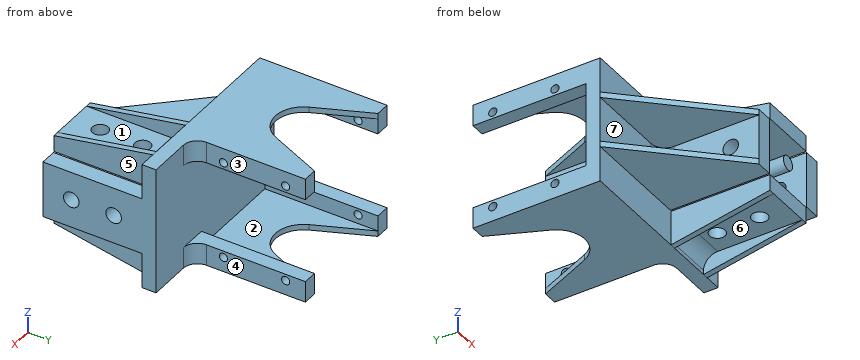
from build123d import *

# Parameters (mm, degrees)
BOSS_EXTRUDE1_DEPTH           = 45
SKETCH3_W                     = 30
SKETCH3_H                     = 40
CUT_EXTRUDE1_DEPTH            = 83.196411114
SKETCH4_W                     = 32
SKETCH4_H                     = 32
SKETCH4_W_2                   = 20.5
SKETCH4_H_2                   = 20.5
SKETCH4_R                     = 2.5
BOSS_EXTRUDE2_DEPTH           = 35
SKETCH6_W                     = 6
SKETCH6_H                     = 6
CUT_EXTRUDE4_DEPTH            = 35
RIB1_REACH                    = 84.092
SKETCH9_WALL_W                = 214.287640152
SKETCH9_WALL_H                = 2
LPATTERN1_COUNT               = 2
LPATTERN1_PITCH               = 18
RIB6_REACH                    = 95.874
SKETCH14_WALL_W               = 225.34562544
SKETCH14_WALL_H               = 2
RIB7_START                    = -2
RIB7_DEPTH                    = 2
CIRPATTERN3_START             = -9.75
CIRPATTERN3_DEPTH             = 2
CIRPATTERN3_START_2           = 8.25
CIRPATTERN3_2_DEPTH           = 2
FILLET2_R                     = 5
FILLET3_R                     = 5
RIB10_REACH                   = 89.794
SKETCH17_WALL_W               = 221.248919868
SKETCH17_WALL_H               = 2
RIB11_REACH                   = 89.794
SKETCH18_WALL_W               = 221.248919868
SKETCH18_WALL_H               = 2
FILLET4_R                     = 10
LPATTERN2_COUNT               = 2
LPATTERN2_PITCH               = 43
FILLET4_OF_LPATTERN2_R        = 10
M5_CLEARANCE_HOLE2_AT_2_COUNT = 2
M5_CLEARANCE_HOLE2_AT_2_PITCH = 15
CIRPATTERN4_START             = 6.5
CIRPATTERN4_OUTLINE_R         = 2.75
CIRPATTERN4_DEPTH             = 5.75
CIRPATTERN4_START_2           = -15.75
CIRPATTERN4_2_OUTLINE_R       = 2.75
CIRPATTERN4_2_DEPTH           = 5.75
CIRPATTERN4_START_3           = 10.5
CIRPATTERN4_3_OUTLINE_R       = 2.75
CIRPATTERN4_3_DEPTH           = 5.75
M2_5_CLEARANCE_HOLE1_D        = 2.9


# Read off the part's stored shape, not the designer's step: Rib7, CirPattern3, CirPattern4
with BuildPart() as part:
    # Sketch2 → Boss-Extrude1 (new body)
    with BuildSketch(Plane.XY):
        Polygon((-48.75, -22.5), (16.25, -22.5), (16.25, -17.5), (-3.75, -17.5), (-3.75, 22.5), (-8.75, 22.5), (-8.75, -17.5), (-43.75, -17.5), (-43.75, 22.5), (-48.75, 22.5), align=None)
    extrude(amount=BOSS_EXTRUDE1_DEPTH)

    # Sketch3 → Cut-Extrude1 (cut, through all)
    with BuildSketch(Plane(origin=(-48.75, 0, 0), x_dir=(0, 0, -1), z_dir=(1, 0, 0))):
        with Locations((-22.5, 2.5)):
            Rectangle(SKETCH3_W, SKETCH3_H)
    extrude(amount=CUT_EXTRUDE1_DEPTH, mode=Mode.SUBTRACT)

    # Sketch4 → Boss-Extrude2 (add)
    # profile 1 of 2: a face of its own
    with BuildSketch(Plane.XZ.offset(22.5)):
        with Locations((0.25, 22.5)):
            Rectangle(SKETCH4_W, SKETCH4_H)
        with Locations((0.25, 22.5)):
            Rectangle(SKETCH4_W_2, SKETCH4_H_2, mode=Mode.SUBTRACT)
    # profile 2 of 2: a face of its own
    with BuildSketch(Plane.XZ.offset(22.5)):
        with Locations(Location((0.25, 22.5, 0), (0, 0, 180))):
            Circle(SKETCH4_R)
    extrude(amount=BOSS_EXTRUDE2_DEPTH)

    # Sketch6 → Cut-Extrude4 (cut)
    with BuildSketch(Plane(origin=(0, -57.5, 0), x_dir=(-1, 0, 0), z_dir=(0, -1, 0))):
        with Locations((12.75, -35.5)):
            Rectangle(SKETCH6_W, SKETCH6_H)
        with Locations((-13.25, -35.5)):
            Rectangle(SKETCH6_W, SKETCH6_H)
        with Locations((-13.25, -9.5)):
            Rectangle(SKETCH6_W, SKETCH6_H)
        with Locations((12.75, -9.5)):
            Rectangle(SKETCH6_W, SKETCH6_H)
    extrude(amount=-CUT_EXTRUDE4_DEPTH, mode=Mode.SUBTRACT)

    # Sketch9 wall → Rib1 (add, up to next)
    with BuildSketch(Plane(origin=(-32.25, -40, 32.5), x_dir=(-0.686012868689, 0.727589406185, 0), z_dir=(-0.727589406185, -0.686012868689, 0)), mode=Mode.PRIVATE) as rib1_sk1:
        with Locations((0, 1)):
            Rectangle(SKETCH9_WALL_W, SKETCH9_WALL_H)
    rib1_tool1 = extrude(rib1_sk1.sketch, amount=-RIB1_REACH, mode=Mode.PRIVATE) - part.part
    rib1 = rib1_tool1.solids().sort_by_distance((-32.25, -40, 32.5))[0]
    add(rib1)

    # LPattern1: Rib1 ×2
    with Locations(*[(0, 0, -i * LPATTERN1_PITCH) for i in range(1, LPATTERN1_COUNT)]):
        add(rib1)

    # Sketch14 wall → Rib6 (add, up to next)
    with BuildSketch(Plane(origin=(10.25, -40, 3.25), x_dir=(0, 0.983188736076, -0.182592193843), z_dir=(0, 0.182592193843, 0.983188736076)), mode=Mode.PRIVATE) as rib6_sk1:
        with Locations((0, 1)):
            Rectangle(SKETCH14_WALL_W, SKETCH14_WALL_H)
    rib6_tool1 = extrude(rib6_sk1.sketch, amount=RIB6_REACH, mode=Mode.PRIVATE) - part.part
    add(rib6_tool1.solids().sort_by_distance((10.25, -40, 3.25))[0])

    # Rib7 outline → Rib7 (add)
    with BuildSketch(Plane.ZY.offset(9.75).offset(RIB7_START)):
        Polygon((0, -22.5), (6.5, -57.5), (6.5, -22.5), align=None)
    extrude(amount=RIB7_DEPTH)

    # CirPattern3 outline → CirPattern3 (add)
    with BuildSketch(Plane.YZ.offset(CIRPATTERN3_START)):
        Polygon((-22.5, 38.5), (-22.5, 45), (-57.5, 38.5), align=None)
    extrude(amount=CIRPATTERN3_DEPTH)

    # CirPattern3 2 outline → CirPattern3 2 (add)
    with BuildSketch(Plane.YZ.offset(CIRPATTERN3_START_2)):
        Polygon((-22.5, 38.5), (-22.5, 45), (-57.5, 38.5), align=None)
    extrude(amount=CIRPATTERN3_2_DEPTH)

    # Fillet2
    fillet2_edges = [part.edges().sort_by_distance(p)[0] for p in [
        (-15.75, -22.5, 22.5),
        (0.25, -22.5, 6.5),
        (0.25, -22.5, 38.5),
    ]]
    fillet(fillet2_edges, radius=FILLET2_R)

    # Fillet3
    fillet3_edges = [part.edges().sort_by_distance(p)[0] for p in [
        (-3.75, -17.5, 41.25),
        (-3.75, -17.5, 3.75),
    ]]
    fillet(fillet3_edges, radius=FILLET3_R)

    # Sketch17 wall → Rib10 (add, up to next)
    with BuildSketch(Plane(origin=(-35, 2.5, 45), x_dir=(0.40081883402, -0.916157334902, 0), z_dir=(0.916157334902, 0.40081883402, 0)), mode=Mode.PRIVATE) as rib10_sk1:
        with Locations((0, 1)):
            Rectangle(SKETCH17_WALL_W, SKETCH17_WALL_H)
    rib10_tool1 = extrude(rib10_sk1.sketch, amount=-RIB10_REACH, mode=Mode.PRIVATE) - part.part
    rib10 = rib10_tool1.solids().sort_by_distance((-35, 2.5, 45))[0]
    add(rib10)

    # Sketch18 wall → Rib11 (add, up to next)
    with BuildSketch(Plane(origin=(-17.5, 2.5, 45), x_dir=(0.40081883402, 0.916157334902, 0), z_dir=(-0.916157334902, 0.40081883402, 0)), mode=Mode.PRIVATE) as rib11_sk1:
        with Locations((0, 1)):
            Rectangle(SKETCH18_WALL_W, SKETCH18_WALL_H)
    rib11_tool1 = extrude(rib11_sk1.sketch, amount=-RIB11_REACH, mode=Mode.PRIVATE) - part.part
    rib11 = rib11_tool1.solids().sort_by_distance((-17.5, 2.5, 45))[0]
    add(rib11)

    # Fillet4
    # the kernel refuses this fillet: 10 mm, written as the material it adds along each edge
    with BuildSketch(Plane(origin=(-26.25, -17.5, 45), x_dir=(-0.4008188340200225, 0.9161573349020514, 0), z_dir=(0, 0, -1))) as fillet4_piece_1:
        with BuildLine():
            CenterArc((FILLET4_R * 2.28571428571, FILLET4_R), FILLET4_R, 137.258755461, 132.741244539)
            Line((FILLET4_R * 1.55128805621, FILLET4_R * 1.67868852459), (0, 0))
            Line((0, 0), (FILLET4_R * 2.28571428571, 0))
        make_face()
    extrude(amount=2)

    # LPattern2: Rib10, Rib11 ×2
    with Locations(*[(0, 0, -i * LPATTERN2_PITCH) for i in range(1, LPATTERN2_COUNT)]):
        add(rib10)
        add(rib11)

    # Fillet4 of LPattern2
    # the kernel refuses this fillet: 10 mm, written as the material it adds along each edge
    with BuildSketch(Plane(origin=(-26.25, -17.5, 59.142857143), x_dir=(-0.4008188340200225, 0.9161573349020515, 0), z_dir=(0, 0, -1))) as fillet4_of_lpattern2_piece_1_section:
        with BuildLine():
            CenterArc((FILLET4_OF_LPATTERN2_R * 2.28571428571, FILLET4_OF_LPATTERN2_R), FILLET4_OF_LPATTERN2_R, 137.258755461, 132.741244539)
            Line((FILLET4_OF_LPATTERN2_R * 1.5512880562, FILLET4_OF_LPATTERN2_R * 1.67868852459), (0, 0))
            Line((0, 0), (FILLET4_OF_LPATTERN2_R * 2.28571428571, 0))
        make_face()
    fillet4_of_lpattern2_piece_1 = extrude(amount=59.142857143, mode=Mode.PRIVATE)
    fillet4_of_lpattern2_piece_1 = split(fillet4_of_lpattern2_piece_1, bisect_by=Plane(origin=(-26.25, -6.732617491, 43), z_dir=(0, 0, 1)), keep=Keep.TOP, mode=Mode.PRIVATE)
    fillet4_of_lpattern2_piece_1 = split(fillet4_of_lpattern2_piece_1, bisect_by=Plane(origin=(-26.25, -6.732617491, 45), z_dir=(0, 0, -1)), keep=Keep.TOP, mode=Mode.PRIVATE)
    add(fillet4_of_lpattern2_piece_1)
    with BuildSketch(Plane(origin=(-26.25, -17.5, 2), x_dir=(-0.4008188340200225, 0.9161573349020514, 0), z_dir=(0, 0, -1))) as fillet4_of_lpattern2_piece_2:
        with BuildLine():
            CenterArc((FILLET4_OF_LPATTERN2_R * 2.28571428571, FILLET4_OF_LPATTERN2_R), FILLET4_OF_LPATTERN2_R, 137.258755461, 132.741244539)
            Line((FILLET4_OF_LPATTERN2_R * 1.55128805621, FILLET4_OF_LPATTERN2_R * 1.67868852459), (0, 0))
            Line((0, 0), (FILLET4_OF_LPATTERN2_R * 2.28571428571, 0))
        make_face()
    extrude(amount=2)

    # Sketch22 → M5 Clearance Hole2 (revolve, cut)
    with BuildSketch(Plane(origin=(0.25, -32.5, 38.5), x_dir=(0, -1, 0), z_dir=(1, 0, 0))):
        Polygon((0, 0), (0, 7.652366702), (2.75, 6), (2.75, 0), align=None)
    m5_clearance_hole2 = revolve(axis=Axis((0.25, -32.5, 44.85), (0, 0, -1)), mode=Mode.SUBTRACT)

    # M5 Clearance Hole2 at 2: M5 Clearance Hole2 ×2
    with Locations(*[(0, -i * M5_CLEARANCE_HOLE2_AT_2_PITCH, 0) for i in range(1, M5_CLEARANCE_HOLE2_AT_2_COUNT)]):
        add(m5_clearance_hole2, mode=Mode.SUBTRACT)

    # CirPattern4 outline → CirPattern4 (cut)
    with BuildSketch(Plane.XY.offset(CIRPATTERN4_START)):
        with Locations((0.25, -47.5)):
            Circle(CIRPATTERN4_OUTLINE_R)
        with Locations((0.25, -32.5)):
            Circle(CIRPATTERN4_OUTLINE_R)
    extrude(amount=CIRPATTERN4_DEPTH, mode=Mode.SUBTRACT)

    # CirPattern4 2 outline → CirPattern4 2 (cut)
    with BuildSketch(Plane.YZ.offset(CIRPATTERN4_START_2)):
        with Locations((-47.5, 22.5)):
            Circle(CIRPATTERN4_2_OUTLINE_R)
        with Locations((-32.5, 22.5)):
            Circle(CIRPATTERN4_2_OUTLINE_R)
    extrude(amount=CIRPATTERN4_2_DEPTH, mode=Mode.SUBTRACT)

    # CirPattern4 3 outline → CirPattern4 3 (cut)
    with BuildSketch(Plane.YZ.offset(CIRPATTERN4_START_3)):
        with Locations((-47.5, 22.5)):
            Circle(CIRPATTERN4_3_OUTLINE_R)
        with Locations((-32.5, 22.5)):
            Circle(CIRPATTERN4_3_OUTLINE_R)
    extrude(amount=CIRPATTERN4_3_DEPTH, mode=Mode.SUBTRACT)

    # M2.5 Clearance Hole1 (through all)
    with Locations(Plane.ZY.offset(48.75)):
        with Locations((5.2, 15.5), (39.8, 15.5), (39.8, -6.5), (5.2, -6.5)):
            Hole(M2_5_CLEARANCE_HOLE1_D / 2)


solid = part.part
The model under review builds one solid part; all positions refer to its coordinate system, in mm. Face numbers are marked on the shaded views. A direction names the side the tool comes from. Coordinates: 2 decimals unless noted, no trailing zeros. Order: outer loops, then holes, each group sorted by start corner. A loop starts at its lowest first (then second) coordinate and runs counter-clockwise, first axis right, second up. Notation, with made-up numbers: (66, 62.25) -> (74, 62.25) arc R23 ccw to (74, 90.25) -> close; hole circle Ø6 at (15.5, -4.5). An arc over 180 degrees is marked (long way). Answer in a Markdown table with one row per item.
(1) Wall thickness on line 1 along Y through (x, z) = (-45.4, 39.8); line 2 along Z through (x, y) = (11.9, -32.5); line 3 along Z through (x, y) = (-15, -6): over which ranges is each line inside the solid? List them lowest first.
Answers:
| item | result |
|---|---|
| line 1 | -22.5 to -7.95, -5.05 to 14.05, 16.95 to 22.5 |
| line 2 | 12.5 to 19.75, 25.25 to 32.5 |
| line 3 | 0 to 2, 43 to 45 |
(2) Consider section C-C (y = -16). Write out the cut boundary in (x, z), plus the area to 3 significant figures.
Answers:
| item | result |
|---|---|
| outline | (-48.75, 0) -> (-2.32, 0) -> (-2.32, 7.5) -> (-8.75, 7.5) -> (-8.75, 2) -> (-43.75, 2) -> (-43.75, 7.5) -> (-48.75, 7.5) -> close; (-48.75, 37.5) -> (-43.75, 37.5) -> (-43.75, 43) -> (-8.75, 43) -> (-8.75, 37.5) -> (-2.32, 37.5) -> (-2.32, 45) -> (-48.75, 45) -> close |
| area | 311 mm² |
(3) Consider section A-A (y = -6.5). State how many separate pieces and enclosed holes the cut face has, plus the area to 3 significant figures.
Answers:
| item | result |
|---|---|
| separate pieces | 6 |
| enclosed holes | 0 |
| area | 232 mm² |
(4) Machinability: for the marked faces 4, 5, 6 and 7, which of the approach directions +Z, -Z, +X, -X, +Y, -Y give a long, thin tool a straight path to every point of the face, cutting with its end or side? Answer none if there is none.
Answers:
| item | result |
|---|---|
| face 4 | +Z, -Z, +X, +Y |
| face 5 | +Z, -Z, +X, -Y |
| face 6 | -Z, -Y |
| face 7 | -X, -Y |
(5) The part is to be moulded in two halves that separate along Z. For the marked faces 1, 2 and 3, say which applies: +Z half, -Z half, draft (parallel to the pull), parting line (faces both ways), or undercut.
Answers:
| item | result |
|---|---|
| face 1 | +Z half |
| face 2 | undercut |
| face 3 | draft |
(6) Consider section B-B (z = 36). Write out the cut boundary in (x, y), plus the area to 3 significant figures.
Answers:
| item | result |
|---|---|
| outline | (-48.75, -22.5) -> (-9.75, -22.5) -> (-9.75, -57.5) -> (10.25, -57.5) -> (10.25, -22.5) -> (16.25, -22.5) -> (16.25, -17.5) -> (-48.75, -17.5) -> close; hole circle Ø5.5 at (0.25, -47.5); hole circle Ø5.5 at (0.25, -32.5) |
| area | 977 mm² |
(7) Consider section D-D (z = 29.5). Write out the cut boundary in (x, y), plus the area to 3 significant figures.
Answers:
| item | result |
|---|---|
| outline | (-48.75, -22.5) -> (-20.75, -22.5) arc R5 cw to (-15.75, -27.5) -> (-15.75, -57.5) -> (-10, -57.5) -> (-10, -22.5) -> (10.5, -22.5) -> (10.5, -57.5) -> (16.25, -57.5) -> (16.25, -17.5) -> (-48.75, -17.5) -> close |
| area | 733 mm² |
(8) Insertion check: pin 1 (3.5 mm diameter, centred on y = -36, z = 39, fed in from +X); pin 2 (0.8 mm diameter, centred on x = 3, z = 44.5, fed in from -Y); pin 3 (1.5 mm diameter, centred on x = -6, z = 20, fed in from +Y). Each pin has a flat end and moves straight along its axis. Give the tip position at first contact, or say it passes through.
Answers:
| item | result |
|---|---|
| pin 1 | x = 10.25 |
| pin 2 | y = -22.5 |
| pin 3 | y = -17.5 |
